from build123d import *

# Parameters (mm, degrees)
F1_DEPTH = 114.3
F2_DEPTH = 120.65
F0_W     = 36.8
F0_H     = 3.8
F3_DEPTH = 111.125
F4_W     = 3.5
F4_H     = 7.7
F5_DEPTH = 4


with BuildPart() as f1:
    # F0 (on Front) → F1 (new body, symmetric)
    with BuildSketch(Plane.XZ):
        Polygon((50.201469934, 10.2439912885), (13.401469934, 10.2439912885), (13.401469934, 8.7439912885), (52.201469934, 8.7439912885), (52.201469934, 10.2439912885), align=None)
        Polygon((13.401469934, 8.7439912885), (13.401469934, 10.2439912885), (-23.398530066, 10.2439912885), (-25.398530066, 10.2439912885), (-25.398530066, 8.7439912885), align=None)
    extrude(amount=F1_DEPTH, both=True)



with BuildPart() as f2:
    # F0 (on Front) → F2 (new body, symmetric)
    with BuildSketch(Plane.XZ):
        Polygon((13.401469934, 15.5439912885), (-27.098530066, 15.5439912885), (-27.098530066, 14.0439912885), (-23.398530066, 14.0439912885), (13.401469934, 14.0439912885), align=None)
        Polygon((53.901469934, 15.5439912885), (13.401469934, 15.5439912885), (13.401469934, 14.0439912885), (50.201469934, 14.0439912885), (53.901469934, 14.0439912885), align=None)
    extrude(amount=F2_DEPTH, both=True)


with BuildPart() as f1_1:
    add(f1.part)

    add(f2.part)  # F3 merges F2
    # F0 (on Front) → F3 (join, symmetric)
    with BuildSketch(Plane.XZ):
        with Locations((-4.998530066, 12.1439912885)):
            Rectangle(F0_W, F0_H)
        with Locations((31.801469934, 12.1439912885)):
            Rectangle(F0_W, F0_H)
    extrude(amount=F3_DEPTH, both=True)

    # F4 (on face) → F5 (join)
    with BuildSketch(Plane(origin=(0, 0, 8.7439912885), x_dir=(1, 0, 0), z_dir=(0, 0, -1))):
        with Locations((-23.648530066, 77.15)):
            Rectangle(F4_W, F4_H)
        with Locations((-27.148530066, 77.15)):
            Rectangle(F4_W, F4_H)
    extrude(amount=F5_DEPTH)


solid = f1_1.part
Design review of the part built by this model. Coordinates are the model's own, in mm. A direction names the side the tool comes from. Give positions to 0.01 mm unless a question says otherwise; leave off trailing zeros. Loops run counter-clockwise (first coordinate to the right, second up) from the corner with the lowest first, then second, coordinate; pieces in that order, holes last. Notation, with made-up numbers: M 8.25,50.25 L 34.25,50.25 A17 ccw 34.25,64.25 Z; hole C 71.25,50 d4. An arc over 180 degrees is marked long. Write item = value, one per line.
Q1. For faces 4 (the flat face through (-21.899, -77, 7)), 5 (the flat face through (-25, -73.3, 7)), 6 (the flat face through (-25, -81, 7)), 7 (the flat face through (-28.899, -77, 7)), list the 3-axis set-ups (+Z, -Z, +X, -X, +Y, -Y) from which the entire face can be reached by the end or side of a thin tool; tool diameter is ignored.
Output values:
face_4 = -Z, +X, +Y, -Y
face_5 = -Z, +X, -X, +Y
face_6 = -Z, +X, -X, -Y
face_7 = +Z, -Z, -X, +Y, -Y
Q2. To check wall thickness, follow line 1 (Z direction, x = 27, y = 87); line 2 (Y direction, x = -22, z = 11) (3 decimals); line 3 (X direction, y = -89.5, z = 13.25). State the ranges of each line that lie inside material, in increasing order. Write a range as [from, to].
Output values:
line_1 = [8.74, 15.54]
line_2 = [-111.125, 111.125]
line_3 = [-23.4, 50.2]
Q3. We need section C-C (z = 7). Give the boundary of the cut face in (x, y).
Output values:
outline = M -28.9,-81 L -21.9,-81 L -21.9,-73.3 L -28.9,-73.3 Z
Q4. Insertion check: pin 1 (1.5 mm diameter, centred on y = 85, z = 10.5, fed in from +X); pin 2 (3 mm diameter, centred on x = -25, z = 6, fed in from +Y); pin 3 (6 mm diameter, centred on x = 18, y = 32, fed in from -Z). Each pin has a flat end and moves straight along its axis. Give the tip position at first contact, or say it passes through.
Output values:
pin_1 = 52.2
pin_2 = -73.3
pin_3 = 8.74
Q5. Draft analysis for pull direction Z (two halves, no side actions). For faces 1 (the flat face through (14, -2, 15.544)), 2 (the flat face through (-24, -1, 10.244)), 3 (the flat face through (-25, -77, 4.744)), state which applies: +Z half, -Z half, draft (parallel to the pull), parting line (faces both ways), or undercut.
Output values:
face_1 = +Z half
face_2 = undercut
face_3 = -Z half
Q6. We need section A-A (x = 16.5). Give the boundary of the cut face in (y, z) (3 decimals).
Output values:
outline = M -120.65,14.044 L -111.125,14.044 L -111.125,10.244 L -114.3,10.244 L -114.3,8.744 L 114.3,8.744 L 114.3,10.244 L 111.125,10.244 L 111.125,14.044 L 120.65,14.044 L 120.65,15.544 L -120.65,15.544 Z
Q7. We need section B-B (y = 58). Give the boundary of the cut face in (x, z), plus the area to 3 significant figures.
Output values:
outline = M -27.1,14.04 L -23.4,14.04 L -23.4,10.24 L -25.4,10.24 L -25.4,8.74 L 52.2,8.74 L 52.2,10.24 L 50.2,10.24 L 50.2,14.04 L 53.9,14.04 L 53.9,15.54 L -27.1,15.54 Z
area = 518 mm^2
